The listing builds one solid part. Answer for the finished solid, in the listing's coordinates (mm). Give positions to 0.01 mm unless a question says otherwise; leave off trailing zeros. Order: outer loops, then holes, each group sorted by start corner. A loop starts at its lowest first (then second) coordinate and runs counter-clockwise, first axis right, second up.
```python
from build123d import *

# Parameters (mm, degrees)
BOSS_EXTRUDE1_START   = 4.175578
SKETCH2_R             = 1.524
BOSS_EXTRUDE1_DEPTH   = 1.285422
CHAMFER1_SIZE         = 0.381
CHAMFER1_SIZE2        = 0.659911358
CHAMFER1_PART_2_SIZE  = 0.381
CHAMFER1_PART_2_SIZE2 = 0.659911358
CHAMFER1_PART_3_SIZE  = 0.381
CHAMFER1_PART_3_SIZE2 = 0.659911358
CHAMFER1_PART_4_SIZE  = 0.381
CHAMFER1_PART_4_SIZE2 = 0.659911358
FILLET1_R             = 0.762


with BuildPart() as part:
    # Sketch1 → Revolve1 (revolve)
    with BuildSketch(Plane.XY, mode=Mode.PRIVATE) as revolve1_sk:
        Polygon((3.302, 0), (3.302, 50.8), (0, 50.8), (0, 53.34), (4.445, 53.34), (4.445, 0), align=None)
    revolve(revolve1_sk.sketch.rotate(Axis((0, 50.8, 0), (0, -1, 0)), 90), axis=Axis((0, 50.8, 0), (0, -1, 0)))  # turned: the seam where the file's is

    # Sketch2 → Boss-Extrude1 (add)
    with BuildSketch(Plane.XY.offset(BOSS_EXTRUDE1_START)):
        with Locations((0, 5.08)):
            Circle(SKETCH2_R)
    boss_extrude1 = extrude(amount=BOSS_EXTRUDE1_DEPTH)

    # Mirror1: Boss-Extrude1 across plane
    add(boss_extrude1.mirror(Plane.XY))

    # Chamfer1
    chamfer1_edges = [part.edges().sort_by_distance(p)[0] for p in [
        (-1.524, 5.08, 5.461),
    ]]
    chamfer1_side = [part.faces().sort_by_distance(p)[0] for p in [
        (-1.524, 5.08, 4.818258203),
    ]]
    chamfer(chamfer1_edges, length=CHAMFER1_SIZE, length2=CHAMFER1_SIZE2, reference=chamfer1_side[0])

    # Chamfer1 part 2
    chamfer1_part_2_edges = [part.edges().sort_by_distance(p)[0] for p in [
        (-1.524, 5.08, -5.461),
    ]]
    chamfer1_part_2_side = [part.faces().sort_by_distance(p)[0] for p in [
        (0, 5.08, -5.461),
    ]]
    chamfer(chamfer1_part_2_edges, length=CHAMFER1_PART_2_SIZE, length2=CHAMFER1_PART_2_SIZE2, reference=chamfer1_part_2_side[0])

    # Chamfer1 part 3
    chamfer1_part_3_edges = [part.edges().sort_by_distance(p)[0] for p in [
        (0, 0, -4.445),
        (0, 0, -3.302),
    ]]
    chamfer1_part_3_side = [part.faces().sort_by_distance(p)[0] for p in [
        (0, 0, -4.319276414),
    ]]
    chamfer(chamfer1_part_3_edges, length=CHAMFER1_PART_3_SIZE, length2=CHAMFER1_PART_3_SIZE2, reference=chamfer1_part_3_side[0])

    # Chamfer1 part 4
    chamfer1_part_4_edges = [part.edges().sort_by_distance(p)[0] for p in [
        (0, 53.34, -4.445),
    ]]
    chamfer1_part_4_side = [part.faces().sort_by_distance(p)[0] for p in [
        (0, 53.34, 0),
    ]]
    chamfer(chamfer1_part_4_edges, length=CHAMFER1_PART_4_SIZE, length2=CHAMFER1_PART_4_SIZE2, reference=chamfer1_part_4_side[0])

    # Fillet1
    fillet1_edges = [part.edges().sort_by_distance(p)[0] for p in [
        (-1.524, 5.08, 4.175577685),
        (-1.524, 5.08, -4.175577685),
    ]]
    fillet(fillet1_edges, radius=FILLET1_R)


solid = part.part
```
1) Find section A-A (z = 0). Write down the section's boundary in (x, y) (3 decimals), then the cut area to 3 significant figures.
Geometry says:
outline: (-4.445, 0.66) - (-4.064, 0) - (-3.683, 0) - (-3.302, 0.66) - (-3.302, 50.8) - (3.302, 50.8) - (3.302, 0.66) - (3.683, 0) - (4.064, 0) - (4.445, 0.66) - (4.445, 52.68) - (4.064, 53.34) - (-4.064, 53.34) - (-4.445, 52.68) - close
area: 138 mm2
2) Find section B-B (y = 12). Write down the section's boundary in (x, z) (3 decimals), then the cut area to 3 significant figures.
Geometry says:
outline: circle Ø8.89 at (0, 0); hole circle Ø6.604 at (0, 0)
area: 27.8 mm2
3) For a pull along X with two mould halves and no side action, classify faces 1 (the flat face through (0, 5, 5.461)), 2 (the cylindrical face through (-0.99, 26.08, 3.15)), 3 (the cylindrical face through (-1.34, 26.31, 4.24)), 4 (the flat face through (0, 50.8, 0)) as +X half, -X half, draft (parallel to the pull), parting line (faces both ways), or undercut.
Geometry says:
face 1: draft
face 2: undercut
face 3: parting line
face 4: undercut
4) Given P1, Ø6, axis at y = 11.5, z = 2, coming from the -X side (3 decimals); P2, Ø1, axis at y = 8.5, z = -3, coming from the +X side; P3, Ø2, axis at x = 1.5, z = -1, coming from the -Y side, each flat-ended and moving along its own axis, determine where each tip first touches the part or whether it passes through.
Geometry says:
P1: stops at x = -4.445
P2: stops at x = 3.68
P3: stops at y = 50.8
5) Straight lines are drawn through the part: probe 1 along X at (y, z) = (35.5, 0) (3 decimals); probe 2 along Y at (x, z) = (1.5, 0.5); probe 3 along Z at (x, y) = (1.5, 9.5). For each, find the intervals that lie inside material, in ascending order.
Geometry says:
probe 1: x = -4.445 to -3.302, 3.302 to 4.445
probe 2: y = 50.8 to 53.34
probe 3: z = -4.18 to -2.94, 2.94 to 4.18
